Model file for the job. Use its own axes, mm. Coordinates: 2 decimals unless noted, no trailing zeros.
Q1. Drill centre lines: probe 1 along X at (y, z) = (-16.25, 157); probe 2 along Z at (x, y) = (784, -17). Where is each one in solid material? Low to high.
Q2. Pull direction Y, two halves, no side cores. Call faces 1 (the flat face through (445, 0, 309)), 2 (the flat face through (445, -9, 609.6)), 3 (the flat face through (445, -19.05, 315)): released by +Y, released by -Y, zero draft, split by the parting line, or undercut.
Q3. Pin check, flat tips, straight feed: P1, Ø5, axis at y = -14, z = 526, coming from the +X side; P2, Ø5, axis at y = -15.5, z = 195.5, coming from the -X side. Stop position of each tip, or through.
from build123d import *

# Parameters (mm, degrees)
F0_W     = 901.7
F0_H     = 609.6
F1_DEPTH = 19.05
F2_W     = 12.7
F2_H     = 6.35
F3_DEPTH = 609.601
F4_W     = 6.35
F4_H     = 12.7
F5_DEPTH = 901.701


with BuildPart() as f1:
    # F0 (on Front) → F1 (new body)
    with BuildSketch(Plane.XZ):
        with Locations((450.85, 304.8)):
            Rectangle(F0_W, F0_H)
    extrude(amount=F1_DEPTH)

    # F2 (on face) → F3 (cut, through all)
    with BuildSketch(Plane.XY.offset(609.6)):
        with Locations((895.35, -15.875)):
            Rectangle(F2_W, F2_H)
        with Locations((6.35, -15.875)):
            Rectangle(F2_W, F2_H)
    extrude(amount=-F3_DEPTH, mode=Mode.SUBTRACT)

    # F4 (on face) → F5 (cut, through all)
    with BuildSketch(Plane.YZ.offset(901.7)):
        with Locations((-15.875, 6.35)):
            Rectangle(F4_W, F4_H)
    extrude(amount=-F5_DEPTH, mode=Mode.SUBTRACT)


solid = f1.part
Answer sheet:
1. probe 1: x = 12.7 to 889
1. probe 2: z = 12.7 to 609.6
2. face 1: released by +Y
2. face 2: zero draft
2. face 3: released by -Y
3. P1: stops at x = 901.7
3. P2: stops at x = 12.7
